Solid Edge part; units mm, degrees
sketch "Sketch1" plane through (0, 0, 0) normal (1, 0, 0) x (0, 1, 0)
  line L0 (0, 0) -> (6, 0)
  line L1 (6, 0) -> (6, 24)
  line L2 (6, 24) -> (12, 30)
  line L3 (12, 30) -> (0, 30)
  line L4 (0, 30) -> (0, 0)
  dimension "D1" = 12
  dimension "D2" = 6
revolve "RevolvedProtrusion1" add sketch "Sketch1" angle 360 about axis through (0, 0, -57) along (0, 0, 1)
sketch "Sketch2" plane through (0, 0, 0) normal (0, -1, 0) x (1, 0, 0)
  line L0 (-1, 32.5562) -> (1, 32.5562)
  line L1 (1, 32.5562) -> (1, 27)
  line L2 (1, 27) -> (-1, 27)
  line L3 (-1, 27) -> (-1, 32.5562)
  dimension "D1" = 1
extrude "Cutout1" cut sketch "Sketch2" along normal mid plane 89.2253
cosmetic_thread "Thread1"
chamfer "Chamfer_3" distance 1 angle 45 1 edges at (-6, 0, 0)
properties part number "6" material "Fe - 410 W"
Geometry: final body of the model. Coordinates: model frame, mm. A direction names the side the tool comes from. Give positions to 0.01 mm unless a question says otherwise; leave off trailing zeros. Order: outer loops, then holes, each group sorted by start corner. A loop starts at its lowest first (then second) coordinate and runs counter-clockwise, first axis right, second up. Notation, with made-up numbers: (-21.75, 19.25) -> (24.25, 19.25) arc R13 cw to (24.25, 35.25) -> close; hole circle Ø1 at (23, 86.5). An arc over 180 degrees is marked (long way). Answer as a JSON object with one key per item and string values.
Q1. First-contact query: pin 1 (5 mm diameter, centred on x = 3.5, z = 12.5, fed in from +Y); pin 2 (5 mm diameter, centred on x = -2, z = 7, fed in from +Y); pin 3 (5 mm diameter, centred on y = -7, z = 23, fed in from -X); pin 4 (1 mm diameter, centred on y = 7, z = 21.5, fed in from +X). Flat tips, straight axial feed; report the tip coordinate or a pass-through.
Entries:
{"pin 1": "stops at y = 5.92", "pin 2": "stops at y = 6", "pin 3": "stops at x = -4.33", "pin 4": "passes through"}
Q2. Access query for faces 1 (the flat face through (0, 0, 27)), 2 (the flat face through (-5, 0, 30)). Directions: +Z, -Z, +X, -X, +Y, -Y. A direction counts if a zero-diameter tool reaches every point of the face in a straight line with its end or side. Return the directions, or none.
Entries:
{"face 1": "+Z, +Y, -Y", "face 2": "+Z, +X, -X, +Y, -Y"}
Q3. Draft query along X for faces 3 (the flat face through (-1, 0, 28)), 4 (the cylindrical face through (0, -6, 13)), 5 (the flat face through (5, 0, 30)). Return one class per face: released by +X, released by -X, zero draft, split by the parting line, or undercut.
Entries:
{"face 3": "undercut", "face 4": "split by the parting line", "face 5": "zero draft"}
Q4. Section C-C (z = 25.5). Output: boundary loops of the cut face in (x, y).
Entries:
{"outline": "circle Ø15 at (0, 0)"}
Q5. Section D-D (z = 6). Output: boundary loops of the cut face in (x, y), plus the area to 3 significant figures.
Entries:
{"outline": "circle Ø12 at (0, 0)", "area": "113 mm^2"}
Q6. Section B-B (x = 0). Output: boundary loops of the cut face in (y, z).
Entries:
{"outline": "(-9, 27) -> (-6, 24) -> (-6, 1) -> (-5, 0) -> (5, 0) -> (6, 1) -> (6, 24) -> (9, 27) -> close"}
Q7. Section A-A (y = 0). Output: boundary loops of the cut face in (x, z), plus the area to 3 significant figures.
Entries:
{"outline": "(-12, 30) -> (-6, 24) -> (-6, 1) -> (-5, 0) -> (5, 0) -> (6, 1) -> (6, 24) -> (12, 30) -> (1, 30) -> (1, 27) -> (-1, 27) -> (-1, 30) -> close", "area": "389 mm^2"}
Q8. Material intervals for probe 1 along X at (y, z) = (0.25, 24); probe 2 along Z at (x, y) = (6.75, -7); probe 3 along Y at (x, z) = (4, 21.5), sorted ascending.
Entries:
{"probe 1": "x = -5.99 to 5.99", "probe 2": "z = 27.72 to 30", "probe 3": "y = -4.47 to 4.47"}
